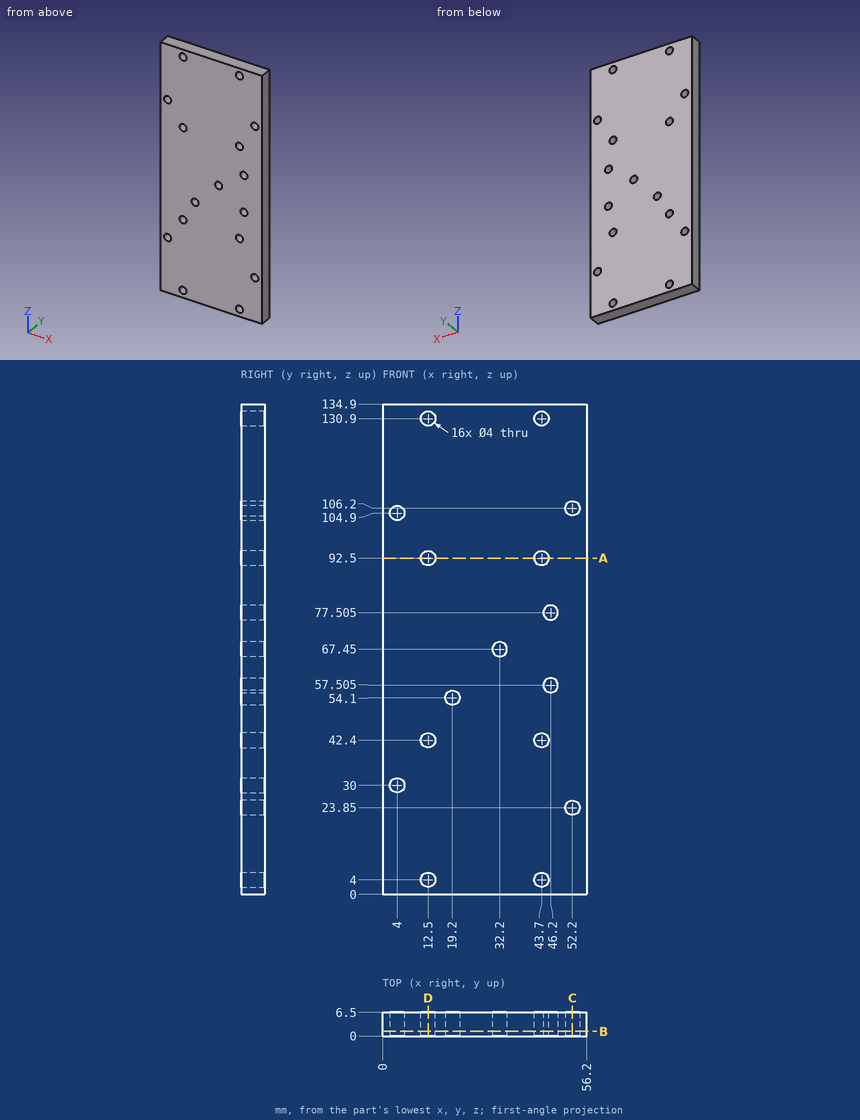
Print and shaded views of the part. All mm, measured from the part's lowest x, y and z. Round coordinates to 2 decimals unless told otherwise and drop trailing zeros. Write each loop counter-clockwise with the first axis right and the second up, starting at its lowest first coordinate (ties: lowest second). Pieces come first, ordered by that corner, then holes. Notation, with made-up numbers: (-29.75, 80.25) -> (-2.75, 80.25) arc R5 ccw to (-2.75, 86.25) -> close; hole circle Ø7 at (19, 37). An arc over 180 degrees is marked (long way). Return JSON: item names as keys, results as strings. Group by question number.
Q1. Saw through at A-A on z = 92.5. Write the cut outline in (x, y).
Q2. Saw through at D-D on x = 12.5. Write the cut outline in (y, z).
Q3. Saw through at B-B on y = 1.25. State how many separate pieces and enclosed holes the cut face has, plus the area to 3 significant figures.
Q4. Probe L1, parallel to X at y = 1.5, z = 92.5; L2, parallel to Z at x = 43.5, y = 1.5; L3, parallel to Z at x = 52.2, y = 3. List the from-to ranges inside material, lowest first. Write a range as [from, to].
Q5. Saw through at C-C on x = 52.2. Write the cut outline in (y, z), plus the area to 3 significant figures.
Answer:
{
 "1": {"outline": "(0, 0) -> (10.5, 0) -> (10.5, 6.5) -> (0, 6.5) -> close; (14.5, 0) -> (41.7, 0) -> (41.7, 6.5) -> (14.5, 6.5) -> close; (45.7, 0) -> (56.2, 0) -> (56.2, 6.5) -> (45.7, 6.5) -> close"},
 "2": {"outline": "(0, 0) -> (6.5, 0) -> (6.5, 2) -> (0, 2) -> close; (0, 6) -> (6.5, 6) -> (6.5, 40.4) -> (0, 40.4) -> close; (0, 44.4) -> (6.5, 44.4) -> (6.5, 90.5) -> (0, 90.5) -> close; (0, 94.5) -> (6.5, 94.5) -> (6.5, 128.9) -> (0, 128.9) -> close; (0, 132.9) -> (6.5, 132.9) -> (6.5, 134.9) -> (0, 134.9) -> close"},
 "3": {"separate pieces": "1", "enclosed holes": "16", "area": "7,380 mm2"},
 "4": {"L1": "[0, 10.5], [14.5, 41.7], [45.7, 56.2]", "L2": "[0, 2.01], [5.99, 40.41], [44.39, 90.51], [94.49, 128.91], [132.89, 134.9]", "L3": "[0, 21.85], [25.85, 104.2], [108.2, 134.9]"},
 "5": {"outline": "(0, 0) -> (6.5, 0) -> (6.5, 21.85) -> (0, 21.85) -> close; (0, 25.85) -> (6.5, 25.85) -> (6.5, 104.2) -> (0, 104.2) -> close; (0, 108.2) -> (6.5, 108.2) -> (6.5, 134.9) -> (0, 134.9) -> close", "area": "825 mm2"}
}
